Verification items for the finished model (mm, model axes). Coordinates: 2 decimals unless noted, no trailing zeros. Write each loop counter-clockwise with the first axis right and the second up, starting at its lowest first coordinate (ties: lowest second). Pieces come first, ordered by that corner, then holes. Notation, with made-up numbers: (54.5, 57.5) -> (71.5, 57.5) arc R12 ccw to (71.5, 70.5) -> close; hole circle Ø4 at (-6, 14). An arc over 180 degrees is marked (long way). Write each question's results on one line, items separated by ' | '. Start each with the question number.
from build123d import *

# Parameters (mm, degrees)
CROQUIS1_R                   = 2.95
SALIENTE_EXTRUIR1_DEPTH      = 1
CORTAR_EXTRUIR1_START        = -0.5
CROQUIS4_R                   = 2.45
CORTAR_EXTRUIR1_DEPTH        = 0.5
SALIENTE_EXTRUIR2_DEPTH      = 18
SALIENTE_EXTRUIR2_DEPTH_BACK = 2
CROQUIS5_R                   = 0.25
CORTAR_EXTRUIR2_START        = -1
CROQUIS6_R                   = 0.25
CORTAR_EXTRUIR2_DEPTH        = 1


with BuildPart() as part:
    # Croquis1 → Saliente-Extruir1 (new body)
    with BuildSketch(Plane(origin=(0, 0, 0), x_dir=(1, 0, 0), z_dir=(0, 1, 0))):
        with Locations(Location((0, 0, 0), (0, 0, 270))):
            Circle(CROQUIS1_R)
    extrude(amount=SALIENTE_EXTRUIR1_DEPTH)

    # Croquis2 → Revolución1 (revolve)
    with BuildSketch(Plane.XY):
        with BuildLine():
            Line((0, 1), (-2.45, 1))
            Line((-2.45, 1), (-2.45, 6.25))
            ThreePointArc((-2.45, 6.25), (-1.732411614, 7.982411614), (0, 8.7))
            Line((0, 8.7), (0, 1))
        make_face()
    revolve(axis=Axis((0, 0, 0), (0, 1, 0)))

    # Croquis4 → Cortar-Extruir1 (cut)
    with BuildSketch(Plane(origin=(0, 0, 0), x_dir=(-1, 0, 0), z_dir=(0, -1, 0)).offset(CORTAR_EXTRUIR1_START)):
        with Locations(Location((0, 0, 0), (0, 0, 90))):
            Circle(CROQUIS4_R)
    extrude(amount=CORTAR_EXTRUIR1_DEPTH, mode=Mode.SUBTRACT)

    # Croquis5 → Saliente-Extruir2 (add, two sides: drawn at the far end of the back side and taken through both)
    with BuildSketch(Plane.XZ.offset(-0.5).offset(-SALIENTE_EXTRUIR2_DEPTH_BACK)):
        with Locations(Location((-1.05, 0, 0), (0, 0, 270))):
            Circle(CROQUIS5_R)
        with Locations(Location((1.05, 0, 0), (0, 0, 270))):
            Circle(CROQUIS5_R)
    extrude(amount=SALIENTE_EXTRUIR2_DEPTH + SALIENTE_EXTRUIR2_DEPTH_BACK)

    # Croquis6 → Cortar-Extruir2 (cut)
    with BuildSketch(Plane.XZ.offset(17.5).offset(CORTAR_EXTRUIR2_START)):
        with Locations(Location((1.05, 0, 0), (0, 0, 270))):
            Circle(CROQUIS6_R)
    extrude(amount=CORTAR_EXTRUIR2_DEPTH, mode=Mode.SUBTRACT)


solid = part.part
1. Sectioned sample at D-D on y = 0.75. Record the cut outline in (x, z), plus the area to 3 significant figures.
2. Depth check by flat-ended pin: pin 1 Ø3 at (x, y) = (0, -12) entering from -Z; pin 2 Ø1 at (x, z) = (-1, -1.5) entering from -Y; pin 3 Ø1.5 at (x, z) = (1.5, -2) entering from -Y. Enter the tip coordinate at first touch or a pass-through.
3. Mould release check, pull along X, two halves, no side actions. Record for faces 1 (the flat face through (0, 0.5, 0)), 2 (the cylindrical face through (0.5, 3.7, -2.4)), 3 (the cylindrical face through (0.736, 0.254, -2.337)): +X half, -X half, draft (parallel to the pull), parting line (faces both ways), or undercut.
4. Sectioned sample at B-B on y = -13.5. Record the cut outline in (x, z).
5. Sectioned sample at A-A on z = 0. Record the cut outline in (x, y).
6. Sectioned sample at C-C on x = -1.05. Record the cut outline in (y, z).
7. Material ranges on probe 1 along X at (y, z) = (0.35, 0); probe 2 along Y at (x, z) = (-2.45, -0.95); probe 3 along Y at (x, z) = (0.1, 0), recorded low to high. Write a range as from..to.
Computed values:
1) outline: circle Ø5.9 at (0, 0) | area: 27.3 mm^2
2) pin 1: stops at z = -0.25 | pin 2: stops at y = 0.5 | pin 3: stops at y = 0
3) face 1: undercut | face 2: parting line | face 3: undercut
4) outline: circle Ø0.5 at (-1.05, 0); circle Ø0.5 at (1.05, 0)
5) outline: (-2.95, 0) -> (-2.45, 0) -> (-2.45, 0.5) -> (-1.3, 0.5) -> (-1.3, -17.5) -> (-0.8, -17.5) -> (-0.8, 0.5) -> (0.8, 0.5) -> (0.8, -16.5) -> (1.3, -16.5) -> (1.3, 0.5) -> (2.45, 0.5) -> (2.45, 0) -> (2.95, 0) -> (2.95, 1) -> (2.45, 1) -> (2.45, 6.25) arc R2.45 ccw to (-2.45, 6.25) -> (-2.45, 1) -> (-2.95, 1) -> close
6) outline: (-17.5, -0.25) -> (0.5, -0.25) -> (0.5, -2.21) -> (0, -2.21) -> (0, -2.76) -> (1, -2.76) -> (1, -2.21) -> (6.25, -2.21) arc R2.21 ccw to (6.25, 2.21) -> (1, 2.21) -> (1, 2.76) -> (0, 2.76) -> (0, 2.21) -> (0.5, 2.21) -> (0.5, 0.25) -> (-17.5, 0.25) -> close
7) probe 1: x = -2.95..-2.45, -1.3..-0.8, 0.8..1.3, 2.45..2.95 | probe 2: y = 0..1 | probe 3: y = 0.5..8.7
